from build123d import *

# Parameters (mm, degrees)
SKETCH1_R                = 1.25
BOSS_EXTRUDE1_DEPTH      = 2
BOSS_EXTRUDE2_DEPTH      = 4
BOSS_EXTRUDE2_DEPTH_BACK = 2
SKETCH2_W                = 29
SKETCH2_H                = 5
FILLET1_R                = 5
SKETCH3_W                = 3
SKETCH3_H                = 6
BOSS_EXTRUDE3_DEPTH      = 8
FILLET2_R                = 2
CUT_EXTRUDE1_DEPTH       = 15
CUT_EXTRUDE1_DEPTH_BACK  = 7
SKETCH4_R                = 1.25


with BuildPart() as part:
    # Sketch1 → Boss-Extrude1 (new body)
    with BuildSketch(Plane(origin=(0, 0, 0), x_dir=(1, 0, 0), z_dir=(0, 1, 0))):
        with BuildLine():
            Line((24.9, 27.6), (25, 27.6))
            ThreePointArc((25, 27.6), (27.828427125, 26.428427125), (29, 23.6))
            Line((29, 23.6), (29, 0))
            Line((29, 0), (0, 0))
            Line((0, 0), (0, 23.6))
            ThreePointArc((0, 23.6), (1.171572875, 26.428427125), (4, 27.6))
            Line((4, 27.6), (4.1, 27.6))
            ThreePointArc((4.1, 27.6), (6.857716447, 26.457716447), (8, 23.7))
            Line((8, 23.7), (8, 3.5))
            Line((8, 3.5), (21, 3.5))
            Line((21, 3.5), (21, 23.7))
            ThreePointArc((21, 23.7), (22.142283553, 26.457716447), (24.9, 27.6))
        make_face()
        with Locations(Location((3.95, 23.6, 0), (0, 0, 270))):
            Circle(SKETCH1_R, mode=Mode.SUBTRACT)
        with Locations(Location((25.05, 23.6, 0), (0, 0, 270))):
            Circle(SKETCH1_R, mode=Mode.SUBTRACT)
        with Locations(Location((25.05, 11, 0), (0, 0, 270))):
            Circle(SKETCH1_R, mode=Mode.SUBTRACT)
        with Locations(Location((3.95, 11, 0), (0, 0, 270))):
            Circle(SKETCH1_R, mode=Mode.SUBTRACT)
    extrude(amount=BOSS_EXTRUDE1_DEPTH)

    # Sketch2 → Boss-Extrude2 (add, two sides: drawn at the far end of the back side and taken through both)
    with BuildSketch(Plane(origin=(0, 2, 0), x_dir=(1, 0, 0), z_dir=(0, 1, 0)).offset(-BOSS_EXTRUDE2_DEPTH_BACK)):
        with Locations((14.5, -2.5)):
            Rectangle(SKETCH2_W, SKETCH2_H)
    extrude(amount=BOSS_EXTRUDE2_DEPTH + BOSS_EXTRUDE2_DEPTH_BACK)

    # Fillet1
    # the kernel refuses this fillet: 5 mm, written as the material it adds along each edge
    with BuildSketch(Plane(origin=(29, 2, 0), x_dir=(0, 0, -1), z_dir=(-1, 0, 0))) as fillet1_piece_1_section:
        with BuildLine():
            CenterArc((4.898979486, -5), FILLET1_R, 90, 78.463040967)
            Line((0, -4), (0, 0))
            Line((0, 0), (4.898979486, 0))
        make_face()
    fillet1_piece_1 = extrude(amount=41.247448714, mode=Mode.PRIVATE)
    fillet1_piece_1 = split(fillet1_piece_1, bisect_by=Plane(origin=(21, 2, 0), z_dir=(1, 0, 0)), keep=Keep.TOP, mode=Mode.PRIVATE)
    add(fillet1_piece_1)
    with BuildSketch(Plane(origin=(41.247448714, 2, 0), x_dir=(0, 0, -1), z_dir=(-1, 0, 0))) as fillet1_piece_2_section:
        with BuildLine():
            CenterArc((4.898979486, -5), FILLET1_R, 90, 78.463040967)
            Line((0, -4), (0, 0))
            Line((0, 0), (4.898979486, 0))
        make_face()
    fillet1_piece_2 = extrude(amount=41.247448714, mode=Mode.PRIVATE)
    fillet1_piece_2 = split(fillet1_piece_2, bisect_by=Plane(origin=(21, 2, 0), z_dir=(-1, 0, 0)), keep=Keep.TOP, mode=Mode.PRIVATE)
    fillet1_piece_2 = split(fillet1_piece_2, bisect_by=Plane(origin=(41.247448714, 2, -3.5), z_dir=(0, 0, 1)), keep=Keep.TOP, mode=Mode.PRIVATE)
    add(fillet1_piece_2)
    with BuildSketch(Plane(origin=(41.247448714, 2, 0), x_dir=(0, 0, -1), z_dir=(-1, 0, 0))) as fillet1_piece_3_section:
        with BuildLine():
            CenterArc((4.898979486, -5), FILLET1_R, 90, 78.463040967)
            Line((0, -4), (0, 0))
            Line((0, 0), (4.898979486, 0))
        make_face()
    fillet1_piece_3 = extrude(amount=41.247448714, mode=Mode.PRIVATE)
    fillet1_piece_3 = split(fillet1_piece_3, bisect_by=Plane(origin=(8, 2, 0), z_dir=(-1, 0, 0)), keep=Keep.TOP, mode=Mode.PRIVATE)
    add(fillet1_piece_3)

    # Sketch3 → Boss-Extrude3 (add)
    with BuildSketch(Plane.XY.offset(5)):
        with Locations((8, 3)):
            Rectangle(SKETCH3_W, SKETCH3_H)
        with Locations((21, 3)):
            Rectangle(SKETCH3_W, SKETCH3_H)
    extrude(amount=BOSS_EXTRUDE3_DEPTH)

    # Fillet2
    fillet2_edges = [part.edges().sort_by_distance(p)[0] for p in [
        (9.5, 3, 5),
        (6.5, 3, 5),
        (19.5, 3, 5),
        (22.5, 3, 5),
    ]]
    fillet(fillet2_edges, radius=FILLET2_R)

    # Sketch4 → Cut-Extrude1 (cut, two sides: drawn at the far end of the back side and taken through both)
    with BuildSketch(Plane(origin=(9.5, 0, 0), x_dir=(0, 0, -1), z_dir=(1, 0, 0)).offset(-CUT_EXTRUDE1_DEPTH_BACK)):
        with Locations(Location((-10, 3, 0), (0, 0, 180))):
            Circle(SKETCH4_R)
    extrude(amount=CUT_EXTRUDE1_DEPTH + CUT_EXTRUDE1_DEPTH_BACK, mode=Mode.SUBTRACT)


solid = part.part
Can you work these out from the model? Positions are in its coordinate system, mm. A direction names the side the tool comes from. Round coordinates to 2 decimals unless told otherwise and drop trailing zeros. Order: outer loops, then holes, each group sorted by start corner. A loop starts at its lowest first (then second) coordinate and runs counter-clockwise, first axis right, second up. Notation, with made-up numbers: (21, 17) - (52, 17) arc R33 cw to (52, 54) - close; hole circle Ø2 at (25.25, -20.5). An arc over 180 degrees is marked (long way). Answer in a Markdown table with one row per item.
(1) Which directions (+Z, -Z, +X, -X, +Y, -Y) give clear straight access to the entire face, cutting with the end or side of a thin tool? Please do faces 1 (the face through (22.112, 0.986, -26.427)), 2 (the face through (6.5, 3, 8.6)), 3 (the face through (9.5, 3, 8.6)), 4 (the face through (27, 3, 5)).
From the geometry:
| item | result |
|---|---|
| face 1 | -Z, +Y, -Y |
| face 2 | +Z, -X, +Y, -Y |
| face 3 | +Z, +Y, -Y |
| face 4 | +Z, +X, +Y, -Y |
(2) Suppose I cut it at C-C, the plane z = -17. Please give me the cut outline in (x, y).
From the geometry:
| item | result |
|---|---|
| outline | (0, 0) - (8, 0) - (8, 2) - (0, 2) - close; (21, 0) - (29, 0) - (29, 2) - (21, 2) - close |
(3) If we mould it in two halves opening along Y, with no side actions, what happens to faces 5 (the face through (23.83, 0.99, -11.27)), 6 (the face through (7.98, 2.95, 8.75)), 7 (the face through (14, 0, -3))? For each: released by +Y, released by -Y, zero draft, split by the parting line, or undercut.
From the geometry:
| item | result |
|---|---|
| face 5 | zero draft |
| face 6 | undercut |
| face 7 | released by -Y |
(4) Suppose I cut it at A-A, the plane z = 10. Please give me the cut outline in (x, y).
From the geometry:
| item | result |
|---|---|
| outline | (6.5, 0) - (9.5, 0) - (9.5, 1.75) - (6.5, 1.75) - close; (6.5, 4.25) - (9.5, 4.25) - (9.5, 6) - (6.5, 6) - close; (19.5, 0) - (22.5, 0) - (22.5, 1.75) - (19.5, 1.75) - close; (19.5, 4.25) - (22.5, 4.25) - (22.5, 6) - (19.5, 6) - close |
(5) Suppose I cut it at B-B, the plane y = 0.75. Please give me the cut outline in (x, z).
From the geometry:
| item | result |
|---|---|
| outline | (0, -23.6) arc R4 ccw to (4, -27.6) - (4.1, -27.6) arc R3.9 ccw to (8, -23.7) - (8, -3.5) - (21, -3.5) - (21, -23.7) arc R3.9 ccw to (24.9, -27.6) - (25, -27.6) arc R4 ccw to (29, -23.6) - (29, 5) - (24.5, 5) arc R2 cw to (22.5, 7) - (22.5, 13) - (19.5, 13) - (19.5, 7) arc R2 cw to (17.5, 5) - (11.5, 5) arc R2 cw to (9.5, 7) - (9.5, 13) - (6.5, 13) - (6.5, 7) arc R2 cw to (4.5, 5) - (0, 5) - close; hole circle Ø2.5 at (3.95, -23.6); hole circle Ø2.5 at (3.95, -11); hole circle Ø2.5 at (25.05, -23.6); hole circle Ø2.5 at (25.05, -11) |
(6) Suppose I cut it at D-D, the plane y = 3. Please give me the cut outline in (x, z).
From the geometry:
| item | result |
|---|---|
| outline | (0, -1.9) - (29, -1.9) - (29, 5) - (24.5, 5) arc R2 cw to (22.5, 7) - (22.5, 8.75) - (19.5, 8.75) - (19.5, 7) arc R2 cw to (17.5, 5) - (11.5, 5) arc R2 cw to (9.5, 7) - (9.5, 8.75) - (6.5, 8.75) - (6.5, 7) arc R2 cw to (4.5, 5) - (0, 5) - close; (6.5, 11.25) - (9.5, 11.25) - (9.5, 13) - (6.5, 13) - close; (19.5, 11.25) - (22.5, 11.25) - (22.5, 13) - (19.5, 13) - close |
(7) For P1, Ø1.3, axis at x = 27, y = 1.5, coming from the +Z side; P2, Ø3, axis at x = 3.95, z = -23.6, coming from the +Y side; P3, Ø1.5, axis at x = 3, y = 2, coming from the -Z side, each with a flat end and sliding along its axis, tell me the tip position at first contact or that it passes through.
From the geometry:
| item | result |
|---|---|
| P1 | stops at z = 5 |
| P2 | stops at y = 2 |
| P3 | stops at z = -27.59 |
(8) Please list where these lines run through material, in increasing order: L1, parallel to X at y = 1.1, z = -23.6; L2, parallel to X at y = 5, z = 8; L3, parallel to X at y = 0.5, z = -6. Write a range as from..to.
From the geometry:
| item | result |
|---|---|
| L1 | x = 0..2.7, 5.2..8, 21..23.8, 26.3..29 |
| L2 | x = 6.5..9.5, 19.5..22.5 |
| L3 | x = 0..8, 21..29 |
